from build123d import *

# Parameters (mm, degrees)
SKETCH_1_W           = 40
SKETCH_1_H           = 20
SKETCH_1_R           = 1.7
SKETCH_1_R_2         = 3
EXTRUDE_1_DEPTH      = 5
SKETCH_2_W           = 5
SKETCH_2_H           = 20
EXTRUDE_2_DEPTH      = 20
EXTRUDE_3_DEPTH      = 1.5
EXTRUDE_3_DEPTH_BACK = 1.5
SKETCH_4_R           = 1.7
CUT_EXTRUDE_1_DEPTH  = 49.218253805
FILLET_1_R           = 3


with BuildPart() as part:
    # 草图1 → 凸台-拉伸1 (new body)
    with BuildSketch(Plane(origin=(0, 0, 0), x_dir=(1, 0, 0), z_dir=(0, 1, 0))):
        Rectangle(SKETCH_1_W, SKETCH_1_H)
        with Locations(Location((4.949747468, 4.949747468, 0), (0, 0, 270))):
            Circle(SKETCH_1_R, mode=Mode.SUBTRACT)
        with Locations(Location((4.949747468, -4.949747468, 0), (0, 0, 270))):
            Circle(SKETCH_1_R, mode=Mode.SUBTRACT)
        with Locations(Location((-4.949747468, -4.949747468, 0), (0, 0, 270))):
            Circle(SKETCH_1_R, mode=Mode.SUBTRACT)
        with Locations(Location((-4.949747468, 4.949747468, 0), (0, 0, 270))):
            Circle(SKETCH_1_R, mode=Mode.SUBTRACT)
        with Locations(Location((0, 0, 0), (0, 0, 270))):
            Circle(SKETCH_1_R_2, mode=Mode.SUBTRACT)
    extrude(amount=EXTRUDE_1_DEPTH)

    # 草图2 → 凸台-拉伸2 (add)
    with BuildSketch(Plane(origin=(0, 5, 0), x_dir=(1, 0, 0), z_dir=(0, 1, 0))):
        with Locations((-17.5, 0)):
            Rectangle(SKETCH_2_W, SKETCH_2_H)
        with Locations((17.5, 0)):
            Rectangle(SKETCH_2_W, SKETCH_2_H)
    extrude(amount=EXTRUDE_2_DEPTH)

    # 草图3 → 凸台-拉伸3 (add, two sides: drawn at the far end of the back side and taken through both)
    with BuildSketch(Plane.XY.offset(-EXTRUDE_3_DEPTH_BACK)):
        Polygon((-15, 20), (-7.5, 5), (-15, 5), align=None)
        Polygon((15, 5), (15, 20), (7.5, 5), align=None)
    extrude(amount=EXTRUDE_3_DEPTH + EXTRUDE_3_DEPTH_BACK)

    # 草图4 → 切除-拉伸1 (cut, through all)
    with BuildSketch(Plane.ZY.offset(20)):
        with Locations((-5, 20)):
            Circle(SKETCH_4_R)
        with Locations((5, 20)):
            Circle(SKETCH_4_R)
        with Locations((5, 10)):
            Circle(SKETCH_4_R)
        with Locations((-5, 10)):
            Circle(SKETCH_4_R)
    extrude(amount=-CUT_EXTRUDE_1_DEPTH, mode=Mode.SUBTRACT)

    # 圆角1
    fillet_1_edges = [part.edges().sort_by_distance(p)[0] for p in [
        (-17.5, 25, 10),
        (-17.5, 25, -10),
        (17.5, 25, -10),
        (17.5, 25, 10),
        (-20, 0, 0),
        (20, 0, 0),
    ]]
    fillet(fillet_1_edges, radius=FILLET_1_R)


solid = part.part
Check sheet for the modelled part. Datum: model origin and axes. Units: mm. A direction names the side the tool comes from. Round coordinates to 2 decimals unless told otherwise and drop trailing zeros. Order: outer loops, then holes, each group sorted by start corner. A loop starts at its lowest first (then second) coordinate and runs counter-clockwise, first axis right, second up. Notation, with made-up numbers: M 29.25,-23.5 L 83.25,-23.5 A19 ccw 83.25,2.5 Z; hole C -0.5,68.5 d2. An arc over 180 degrees is marked long. One line per item, written item: value. Start each with the question number.
1. Section check D-D on y = 6.25. Enter the section's corners in (x, z) (3 decimals).
2. Gauge pin test, flat ends, axial feed: P1, Ø2, axis at x = 13, y = 13, coming from the -Z side; P2, Ø10, axis at x = 4, z = 0, coming from the +Y side; P3, Ø4.5, axis at x = -4.95, z = 4.95, coming from the +Y side. Record the tip position at first contact, or that the pin passes through.
3. Section check A-A on y = 10. Give the number of separate pieces and of enclosed holes in the cut face, and give its area (3 significant figures).
4. Release check for a two-part mould opening along X. For faces 1 (the cylindrical face through (19.1, 0.86, -0.14)), 2 (the cylindrical face through (17.5, 8.5, -4.2)), 3 (the flat face through (13, 9, -1.5)), 4 (the cylindrical face through (-5.6, 2.46, 6.52)) record: released by +X, released by -X, zero draft, split by the parting line, or undercut.
5. Access from +Z, -Z, +X, -X, +Y, -Y to the whole of each face (thin tool, end or side, straight path). Record for faces 5 (the cylindrical face through (-17.535, 21.433, 5.914)), 6 (the flat face through (-13, 9, -1.5)), 7 (the flat face through (-4, 5, 0)), 8 (the flat face through (-11.3, 12.6, 0)), 9 (the cylindrical face through (17.54, 24.1, -9.14)).
6. Section check B-B on z = 0. Enter the section's corners in (x, y).
7. Scan lines: line 1 along X through (y, z) = (5.25, -7); line 2 along Z through (x, y) = (-4.5, 3); line 3 along Y through (x, z) = (9, -3.5). Record each from-to range of solid material in increasing order.
8. Section check C-C on x = 0. Enter the section's corners in (y, z), and give its area (3 significant figures).
Results found:
1. outline: M -20,-10 L -15,-10 L -15,-1.5 L -8.125,-1.5 L -8.125,1.5 L -15,1.5 L -15,10 L -20,10 Z; M 8.125,-1.5 L 15,-1.5 L 15,-10 L 20,-10 L 20,10 L 15,10 L 15,1.5 L 8.125,1.5 Z
2. P1: z = -1.5
2. P2: y = 8
2. P3: y = 5
3. separate pieces: 6
3. enclosed holes: 0
3. area: 162 mm^2
4. face 1: released by +X
4. face 2: zero draft
4. face 3: undercut
4. face 4: undercut
5. face 5: +X, -X
5. face 6: -Z, +Y
5. face 7: +Y
5. face 8: +Z, -Z, +Y
5. face 9: -Z, +X, -X, +Y
6. outline: M -20,3 A3 ccw -17,0 L -3,0 L -3,5 L -7.5,5 L -15,20 L -15,25 L -20,25 Z; M 3,0 L 17,0 A3 ccw 20,3 L 20,25 L 15,25 L 15,20 L 7.5,5 L 3,5 Z
7. line 1: -20 to -15, 15 to 20
7. line 2: -10 to -6.59, -3.31 to 3.31, 6.59 to 10
7. line 3: 0 to 5
8. outline: M 0,-10 L 5,-10 L 5,-3 L 0,-3 Z; M 0,3 L 5,3 L 5,10 L 0,10 Z
8. area: 70.0 mm^2
